Autodesk Inventor part; units mm, degrees
ref_plane "YZ Plane" through (0, 0, 0) normal (1, 0, 0) x (0, 1, 0)
ref_plane "XZ Plane" through (0, 0, 0) normal (0, 1, 0) x (-1, 0, 0)
ref_plane "XY Plane" through (0, 0, 0) normal (0, 0, 1) x (1, 0, 0)
sketch "Náčrt1" plane through (0, 0, 0) normal (0, 0, 1) x (1, 0, 0)
  arc A0 (3, -31.8591) -> (-3, -31.8591) centre (0, 0) ccw
  circle A1 centre (100, 0) radius 12.5
  arc A2 (75.5051, -5) -> (75.5051, 5) centre (100, 0) ccw
  line L0 (12.5, 48.4123) -> (106.25, 24.2061)
  line L1 (49.7494, 5) -> (75.5051, 5)
  line L2 (75.5051, -5) -> (49.7494, -5)
  line L3 (3, -75) -> (25, -75)
  line L4 (-3, -75) -> (-25, -75)
  line L5 (-25, -75) -> (-25, -43.3013)
  line L6 (25, -75) -> (25, -43.3013)
  line L7 (3, -75) -> (3, -31.8591)
  line L8 (-3, -75) -> (-3, -31.8591)
  arc A3 (25, -43.3013) -> (49.7494, -5) centre (0, 0) ccw
  arc A4 (49.7494, 5) -> (-25, -43.3013) centre (0, 0) ccw
  dimension "d1" = 64
  dimension "d3" = 25
  dimension "d4" = 50
  dimension "d9" = 10
  dimension "d10" = 22
  dimension "d11" = 22
  dimension "d12" = 6
extrude "Vysunutí1" add sketch "Náčrt1" against normal blind 20 contours A0 L8 L4 L5 A4 L1 A2 L2 A3 L6 L3 L7
extrude "Vysunutí2" add sketch "Náčrt1" against normal blind 5 contours L0 A2 L1 A4
extrude "Vysunutí3" add sketch "Náčrt1" along normal blind 5 contours L0 A2 L1 A4
extrude "Vysunutí4" add sketch "Náčrt1" along normal blind 20 contours A0 L8 L4 L5 A4 L1 A2 L2 A3 L6 L3 L7
sketch "Náčrt2" plane through (25, -75, -20) normal (1, 0, 0) x (0, 0, -1)
  point P0 (-20, 75)
  point P1 (-18.8172, 13.7965)
hole "Díra1" at (25, -61.2035, -1.1828) direction (-1, 0, 0) diameter 15 end through all
properties part number "5"
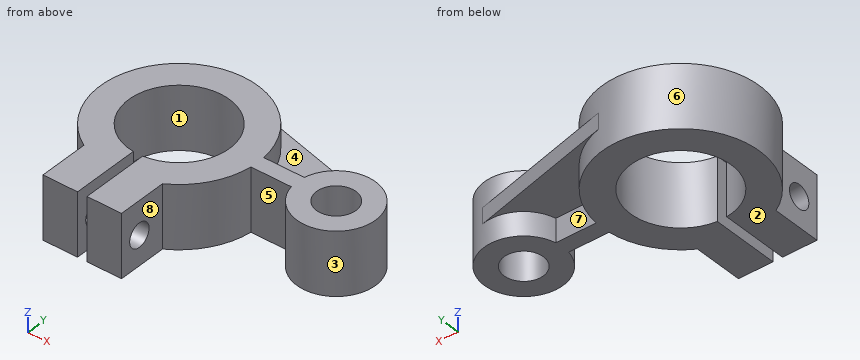
Work out the finished part from the listing and answer in its coordinate system (mm). Face numbers are marked on the shaded views. A direction names the side the tool comes from. Coordinates: 2 decimals unless noted, no trailing zeros. Write each loop counter-clockwise with the first axis right and the second up, starting at its lowest first coordinate (ties: lowest second). Pieces come first, ordered by that corner, then holes.
1. The part is cut by section C-C, the plane z = 10. Write down the section's boundary in (x, y).
Results list:
outline: (-25, -75) - (-3, -75) - (-3, -31.86) arc R32 cw (long way) to (3, -31.86) - (3, -75) - (25, -75) - (25, -43.3) arc R50 ccw to (49.75, -5) - (75.51, -5) arc R25 ccw (long way) to (75.51, 5) - (49.75, 5) arc R50 ccw (long way) to (-25, -43.3) - close; hole circle Ø25 at (100, 0)
2. The part is cut by section B-B, the plane y = 0. Write down the section's boundary in (x, z), and give its area (3 significant figures).
Results list:
outline: (-50, -20) - (-32, -20) - (-32, 20) - (-50, 20) - close; (32, -20) - (87.5, -20) - (87.5, 20) - (32, 20) - close; (112.5, -20) - (125, -20) - (125, 20) - (112.5, 20) - close
area: 3,440 mm2
3. The part is cut by section A-A, the plane y = -46. Write down the section's boundary in (x, z), and give its area (3 significant figures).
Results list:
outline: (-25, -20) - (-3, -20) - (-3, 20) - (-25, 20) - close; (3, -20) - (25, -20) - (25, 20) - (3, 20) - close
area: 1,760 mm2
4. Consider line 1 along X through (y, z) = (-1, -16.5); line 2 along X through (y, z) = (9, 10.5); line 3 along Z through (x, y) = (93.5, 25). Determine where each line is inside the solid, lowest interval first.
Results list:
line 1: x = -49.99 to -31.98, 31.98 to 87.54, 112.46 to 124.98
line 2: x = -49.18 to -30.71, 30.71 to 49.18, 76.68 to 91.33, 108.67 to 123.32
line 3: z = -5 to 5
5. The part is cut by section D-D, the plane x = 93.5. Write down the section's boundary in (y, z).
Results list:
outline: (-24.14, -20) - (-10.68, -20) - (-10.68, 20) - (-24.14, 20) - close; (10.68, -20) - (24.14, -20) - (24.14, -5) - (27.5, -5) - (27.5, 5) - (24.14, 5) - (24.14, 20) - (10.68, 20) - close
6. For the marked faces 4, 5, 6, 7 and 8, determine the directions among +Z, -Z, +X, -X, +Y, -Y from which every point of the face is accessible in a straight line to the end or side of a thin tool.
Results list:
face 4: +Z, +Y
face 5: +Z, -Z, -Y
face 6: none
face 7: -Z, +Y
face 8: +Z, -Z, +X, -Y
7. For a pull along Y with two mould halves and no side action, classify the marked faces 1, 2 and 3 as +Y half, -Y half, draft (parallel to the pull), parting line (faces both ways), or undercut.
Results list:
face 1: undercut
face 2: draft
face 3: parting line
8. Flat-ended cylindrical pins translate along their axes: pin 1 (19.5 mm diameter, centred on y = -61.2, z = -1.18, fed in from +X); pin 2 (6 mm diameter, centred on x = 72, z = -3, fed in from +Y); pin 3 (2 mm diameter, centred on y = -42.5, z = 0.5, fed in from -X). Find the tip coordinate at first contact, or state that the pin passes through.
Results list:
pin 1: stops at x = 25
pin 2: stops at y = 33.82
pin 3: stops at x = -27.89
